from build123d import *

# Parameters (mm, degrees)
SKETCH_1_W          = 65
SKETCH_1_H          = 15
EXTRUDE_1_DEPTH     = 2
SKETCH_2_R          = 1.25
SKETCH_2_R_2        = 3.45
SKETCH_2_R_3        = 1.5
SKETCH_2_R_4        = 1
CUT_EXTRUDE_1_DEPTH = 2
SKETCH_4_R          = 1.5
EXTRUDE_2_DEPTH     = 2
SKETCH_5_R          = 7.5
SKETCH_5_R_2        = 7.1
EXTRUDE_3_DEPTH     = 8
EXTRUDE_START       = -8
SKETCH_5_5_R        = 1.25
SKETCH_5_5_R_2      = 7.1
SKETCH_5_5_R_3      = 1
SKETCH_5_5_R_4      = 1.5
EXTRUDE_4_DEPTH     = 6
CUT_EXTRUDE_START   = -5.5
SKETCH_5_6_R        = 1.25
SKETCH_5_6_R_2      = 7.1
CUT_EXTRUDE_3_DEPTH = 5.5


with BuildPart() as part:
    # 草图1 → 凸台-拉伸1 (new body)
    with BuildSketch(Plane(origin=(0, 0, 0), x_dir=(1, 0, 0), z_dir=(0, 1, 0))):
        with Locations((-7.5, 0)):
            Rectangle(SKETCH_1_W, SKETCH_1_H)
    extrude(amount=EXTRUDE_1_DEPTH)

    # 草图2 → 切除-拉伸1 (cut)
    with BuildSketch(Plane(origin=(0, 0, 0), x_dir=(1, 0, 0), z_dir=(0, 1, 0))):
        with Locations(Location((0, 0, 0), (0, 0, 270))):
            Circle(SKETCH_2_R)
        with Locations(Location((-16, 0, 0), (0, 0, 90))):
            Circle(SKETCH_2_R_2)
        with Locations(Location((-32, 0, 0), (0, 0, 270))):
            Circle(SKETCH_2_R_3)
        with Locations(Location((-26.5, 0, 0), (0, 0, 270))):
            Circle(SKETCH_2_R_4)
        with Locations(Location((-32, -5.5, 0), (0, 0, 270))):
            Circle(SKETCH_2_R_4)
        with Locations(Location((-37.5, 0, 0), (0, 0, 270))):
            Circle(SKETCH_2_R_4)
        with Locations(Location((-32, 5.5, 0), (0, 0, 270))):
            Circle(SKETCH_2_R_4)
    extrude(amount=CUT_EXTRUDE_1_DEPTH, mode=Mode.SUBTRACT)

    # 草图4 → 凸台-拉伸2 (add)
    with BuildSketch(Plane.XY.offset(7.5)):
        with Locations(Location((20, 1, 0), (0, 0, 221.810314896))):
            Circle(SKETCH_4_R)
        with Locations(Location((-20, 1, 0), (0, 0, 221.810314896))):
            Circle(SKETCH_4_R)
    extrude(amount=EXTRUDE_2_DEPTH)

    # 草图5 → 凸台-拉伸3 (add)
    # profile 1 of 2: a face of its own
    with BuildSketch(Plane(origin=(0, 2, 0), x_dir=(1, 0, 0), z_dir=(0, 1, 0))):
        with Locations(Location((-32, 0, 0), (0, 0, 270))):
            Circle(SKETCH_5_R)
        with Locations(Location((-32, 0, 0), (0, 0, 270))):
            Circle(SKETCH_5_R_2, mode=Mode.SUBTRACT)
    # profile 2 of 2: a face of its own
    with BuildSketch(Plane(origin=(0, 2, 0), x_dir=(1, 0, 0), z_dir=(0, 1, 0))):
        with BuildLine():
            Line((5.149029035, -6.7), (-5.149029035, -6.7))
            ThreePointArc((-5.149029035, -6.7), (-8.45, 0), (-5.149029035, 6.7))
            Line((-5.149029035, 6.7), (5.149029035, 6.7))
            ThreePointArc((5.149029035, 6.7), (8.45, 0), (5.149029035, -6.7))
        make_face()
        with BuildLine():
            Line((4.905354218, -6), (-4.905354218, -6))
            ThreePointArc((-4.905354218, -6), (-7.75, 0), (-4.905354218, 6))
            Line((-4.905354218, 6), (4.905354218, 6))
            ThreePointArc((4.905354218, 6), (7.75, 0), (4.905354218, -6))
        make_face(mode=Mode.SUBTRACT)
    extrude(amount=-EXTRUDE_3_DEPTH)

    # 草图5<5> → 凸台-拉伸4 (add)
    # profile 1 of 2: a face of its own
    with BuildSketch(Plane(origin=(0, 2, 0), x_dir=(1, 0, 0), z_dir=(0, 1, 0)).offset(EXTRUDE_START)):
        with BuildLine():
            Line((4.905354218, -6), (-4.905354218, -6))
            ThreePointArc((-4.905354218, -6), (-7.75, 0), (-4.905354218, 6))
            Line((-4.905354218, 6), (4.905354218, 6))
            ThreePointArc((4.905354218, 6), (7.75, 0), (4.905354218, -6))
        make_face()
        with Locations(Location((0, 0, 0), (0, 0, 270))):
            Circle(SKETCH_5_5_R, mode=Mode.SUBTRACT)
    # profile 2 of 2: a face of its own
    with BuildSketch(Plane(origin=(0, 2, 0), x_dir=(1, 0, 0), z_dir=(0, 1, 0)).offset(EXTRUDE_START)):
        with Locations((-32, 0)):
            Circle(SKETCH_5_5_R_2)
        with Locations(Location((-32, 5.5, 0), (0, 0, 270))):
            Circle(SKETCH_5_5_R_3, mode=Mode.SUBTRACT)
        with Locations(Location((-37.5, 0, 0), (0, 0, 270))):
            Circle(SKETCH_5_5_R_3, mode=Mode.SUBTRACT)
        with Locations(Location((-32, 0, 0), (0, 0, 270))):
            Circle(SKETCH_5_5_R_4, mode=Mode.SUBTRACT)
        with Locations(Location((-26.5, 0, 0), (0, 0, 270))):
            Circle(SKETCH_5_5_R_3, mode=Mode.SUBTRACT)
        with Locations(Location((-32, -5.5, 0), (0, 0, 270))):
            Circle(SKETCH_5_5_R_3, mode=Mode.SUBTRACT)
    extrude(amount=EXTRUDE_4_DEPTH)

    # 草图5<6> → 切除-拉伸3 (cut)
    # profile 1 of 2: a face of its own
    with BuildSketch(Plane(origin=(0, 2, 0), x_dir=(1, 0, 0), z_dir=(0, 1, 0)).offset(CUT_EXTRUDE_START)):
        with BuildLine():
            Line((4.905354218, -6), (-4.905354218, -6))
            ThreePointArc((-4.905354218, -6), (-7.75, 0), (-4.905354218, 6))
            Line((-4.905354218, 6), (4.905354218, 6))
            ThreePointArc((4.905354218, 6), (7.75, 0), (4.905354218, -6))
        make_face()
        with Locations(Location((0, 0, 0), (0, 0, 270))):
            Circle(SKETCH_5_6_R, mode=Mode.SUBTRACT)
    # profile 2 of 2: a face of its own
    with BuildSketch(Plane(origin=(0, 2, 0), x_dir=(1, 0, 0), z_dir=(0, 1, 0)).offset(CUT_EXTRUDE_START)):
        with Locations(Location((-32, 0, 0), (0, 0, 270))):
            Circle(SKETCH_5_6_R_2)
    extrude(amount=CUT_EXTRUDE_3_DEPTH, mode=Mode.SUBTRACT)


solid = part.part
Geometry check sheet. Reference: the model listing, model coordinates, mm. A direction names the side the tool comes from. Round coordinates to 2 decimals unless told otherwise and drop trailing zeros. Order: outer loops, then holes, each group sorted by start corner. A loop starts at its lowest first (then second) coordinate and runs counter-clockwise, first axis right, second up. Notation, with made-up numbers: (70.25, 89) - (110.25, 89) arc R28 ccw to (110.25, 118) - close; hole circle Ø5 at (75.5, -2). An arc over 180 degrees is marked (long way). One line per question, with ' | ' between items. Start each with the question number.
(1) Sectioned sample at D-D on z = -2.5. Record the cut outline in (x, y), and give its area (3 significant figures).
(2) Sectioned sample at C-C on y = -4.75. Record the cut outline in (x, z).
(3) Release check for a two-part mould opening along X. For faces 1 (the cylindrical face through (8.45, -2.96, -0.11)), 2 (the cylindrical face through (-1.22, -4.77, -0.27)), 3 (the flat face through (-39.6, 0, -1.7)) record: released by +X, released by -X, zero draft, split by the parting line, or undercut.
(4) Sectioned sample at A-A on y = -2.25. Record the cut outline in (x, z), and give its area (3 significant figures).
(5) Depth check by flat-ended pin: pin 1 Ø4.5 at (x, z) = (-10, -1.5) entering from +Y; pin 2 Ø1 at (x, y) = (23.5, 1) entering from +Z; pin 3 Ø3.5 at (x, z) = (1.5, 0) entering from +Y. Enter the tip coordinate at first touch or a pass-through.
(6) Thickness scan on L1, parallel to X at y = -3, z = -1.5; L2, parallel to Z at x = -32, y = -4.85; L3, parallel to X at y = -3.25, z = 1.25. Record the ranges inside material, lowest first. Write a range as [from, to].
(7) Sectioned sample at B-B on x = -16. Record the cut outline in (y, z), and give its area (3 significant figures).
(8) Access from +Z, -Z, +X, -X, +Y, -Y to the whole of each face (thin tool, end or side, straight path). Record for faces 4 (the cylindrical face through (-8.45, -2.96, 0.11)), 5 (the flat face through (-30, -3.5, 0)), 6 (the flat face through (0, -3, 6.7)), 7 (the flat face through (-8, 2, 0)), 8 (the cylindrical face through (-18.5, 1, 8.5)).
Conclusion:
1) outline: (-40, 0) - (-39.07, 0) - (-39.07, -6) - (-24.93, -6) - (-24.93, 0) - (-18.38, 0) - (-18.38, 2) - (-25.35, 2) - (-25.35, -3.5) - (-38.65, -3.5) - (-38.65, 2) - (-40, 2) - close; (-13.62, 0) - (-8.07, 0) - (-8.07, -6) - (8.07, -6) - (8.07, 0) - (25, 0) - (25, 2) - (7.34, 2) - (7.34, -3.5) - (-7.34, -3.5) - (-7.34, 2) - (-13.62, 2) - close | area: 148 mm2
2) outline: circle Ø15 at (-32, 0); (-5.15, -6.7) - (5.15, -6.7) arc R8.45 ccw to (5.15, 6.7) - (-5.15, 6.7) arc R8.45 ccw to start; hole circle Ø2 at (-37.5, 0); hole circle Ø3 at (-32, 0); hole circle Ø2 at (-32, -5.5); hole circle Ø2 at (-32, 5.5); hole circle Ø2 at (-26.5, 0); hole circle Ø2.5 at (0, 0)
3) face 1: released by +X | face 2: undercut | face 3: zero draft
4) outline: circle Ø15 at (-32, 0); (-5.15, -6.7) - (5.15, -6.7) arc R8.45 ccw to (5.15, 6.7) - (-5.15, 6.7) arc R8.45 ccw to start; hole circle Ø14.2 at (-32, 0); hole (-4.91, -6) - (4.91, -6) arc R7.75 ccw to (4.91, 6) - (-4.91, 6) arc R7.75 ccw to start | area: 52.9 mm2
5) pin 1: stops at y = 2 | pin 2: stops at z = 7.5 | pin 3: stops at y = -3.5
6) L1: x = [-39.35, -38.94], [-25.06, -24.65], [-8.32, -7.6], [7.6, 8.32] | L2: z = [-7.5, -6.5], [-4.5, -1.5], [1.5, 4.5], [6.5, 7.5] | L3: x = [-39.4, -38.99], [-25.01, -24.6], [-8.36, -7.65], [7.65, 8.36]
7) outline: (0, -7.5) - (2, -7.5) - (2, -3.45) - (0, -3.45) - close; (0, 3.45) - (2, 3.45) - (2, 7.5) - (0, 7.5) - close | area: 16.2 mm2
8) face 4: -Y | face 5: +Y | face 6: +Z, +X, -Y | face 7: -Z, +X, -X, +Y | face 8: +Z
